Check sheet for the modelled part. Datum: model origin and axes. Units: mm. Face numbers are marked on the shaded views. A direction names the side the tool comes from. Round coordinates to 2 decimals unless told otherwise and drop trailing zeros. Write each loop counter-clockwise with the first axis right and the second up, starting at its lowest first coordinate (ties: lowest second). Pieces come first, ordered by that corner, then holes. Notation, with made-up numbers: (3, 47) -> (31, 47) arc R28 cw to (31, 85) -> close; hole circle Ø5 at (28, -30.75). An arc over 180 degrees is marked (long way). Answer as a JSON object with one key per item and string values. Group by question number.
```python
from build123d import *

# Parameters (mm, degrees)
F0_W           = 76.2
F0_H           = 127
F0_W_2         = 63.5
F0_H_2         = 114.3
F1_DEPTH       = 762
F2_R           = 19.05
F3_DEPTH       = 12.7
F9_W           = 50.8
F9_H           = 127
F9_W_2         = 38.1
F9_H_2         = 114.3
F10_DEPTH      = 381
F12_DEPTH      = 9.525
F12_DEPTH_BACK = 0.254


with BuildPart() as f1:
    # F0 (on Front) → F1 (new body, symmetric)
    with BuildSketch(Plane.XZ):
        with Locations((38.1, 0)):
            Rectangle(F0_W, F0_H)
        with Locations((38.1, 0)):
            Rectangle(F0_W_2, F0_H_2, mode=Mode.SUBTRACT)
    extrude(amount=F1_DEPTH, both=True)

    # F2 (on face) → F3 (join)
    with BuildSketch(Plane.XY.offset(63.5)):
        with BuildLine():
            ThreePointArc((-11.159232, 827.040768), (-65.040768, 827.040768), (-65.040768, 773.159232))
            Line((-65.040768, 773.159232), (11.159232, 696.959232))
            ThreePointArc((11.159232, 696.959232), (65.040768, 696.959232), (65.040768, 750.840768))
            Line((65.040768, 750.840768), (-11.159232, 827.040768))
        make_face()
        with Locations((-38.1, 800.1)):
            Circle(F2_R, mode=Mode.SUBTRACT)
    extrude(amount=F3_DEPTH)

    # F4: F1 across plane


with BuildPart() as f1_1:
    add(f1.part)
    add(f1.part.mirror(Plane.XY))

    # F9 (on face) → F10 (join)
    with BuildSketch(Plane(origin=(-10.770568, 0, 40.196307), x_dir=(0.965926, 0, 0.258819), z_dir=(-0.258819, 0, 0.965926))):
        with Locations((51.938557, 0)):
            Rectangle(F9_W, F9_H)
        with Locations((51.938557, 0)):
            Rectangle(F9_W_2, F9_H_2, mode=Mode.SUBTRACT)
    extrude(amount=F10_DEPTH)

    # F11 (on face) → F12 (join, two sides)
    with BuildSketch(Plane(origin=(74.70331, 0, 20.016692), x_dir=(0, 1, 0), z_dir=(0.965926, 0, 0.258819))) as f12_sk:
        Polygon((0, 422.614279), (-63.5, 422.614279), (-602.764468, 45.017233), (-381.346724, 45.017233), (0, 312.039085), align=None)
    extrude(amount=F12_DEPTH)
    extrude(f12_sk.sketch, amount=-F12_DEPTH_BACK)

    # F13: F1 across face


with BuildPart() as f1_2:
    add(f1_1.part)
    add(f1_1.part.mirror(Plane(origin=(-15.767609, 0, 376.059646), x_dir=(-1, 0, 0), z_dir=(0, 1, 0))))


solid = f1_2.part
```
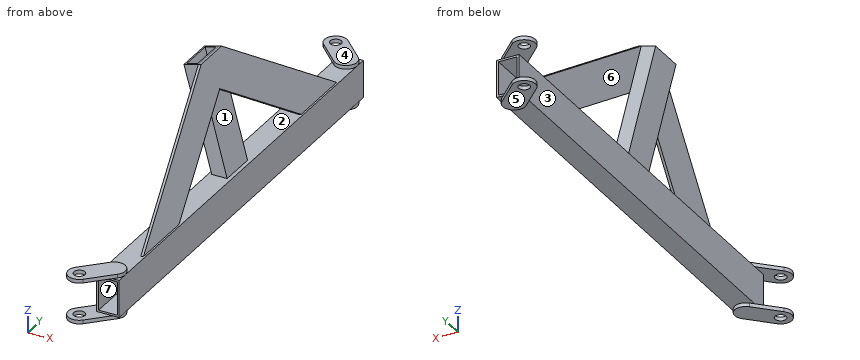
(1) Go/stop test with flat-tipped pins: pin 1 Ø1 at (x, y) = (-2, 400.5) entering from -Z; pin 2 Ø2.5 at (x, z) = (32.5, 51) entering from -Y; pin 3 Ø3 at (x, z) = (29.5, 54.5) entering from +Y; pin 4 Ø4 at (x, y) = (17.5, -357) entering from +Z. Record where each tip stops, or that it passes through.
(2) Section check D-D on x = 38.1. State how many separate pieces and enclosed holes the cut face has, then the cut area to 3 significant figures.
(3) Access from +Z, -Z, +X, -X, +Y, -Y to the whole of each face (thin tool, end or side, straight path). Record for the marked faces 4, 5, 6 and 7.
(4) Section check C-C on y = -639.5. Record the cut outline in (x, z), then the cut area to 3 significant figures.
(5) Release check for a two-part mould opening along Y. For the marked faces 1, 2 and 3 record: pulls with the +Y half, pulls with the -Y half, needs draft (parallel to the pull), parting line crosses it, or undercut.
(6) Scan lines: line 1 along Z through (x, y) = (7, -490); line 2 along X through (y, z) = (-454, -32); line 3 along Y through (x, z) = (-38.1, -69). Record each from-to range of solid material in increasing order.
(7) Section check A-A on z = 161.5. Record the cut outline in (x, y), then the cut area to 3 significant figures.
(8) Section check B-B on z = -23.5. Record the cut outline in (x, y), then the cut area to 3 significant figures.
Data:
{
 "1": {"pin 1": "passes through", "pin 2": "stops at y = -63.5", "pin 3": "stops at y = 63.5", "pin 4": "stops at z = 231"},
 "2": {"separate pieces": "4", "enclosed holes": "1", "area": "44,800 mm²"},
 "3": {"face 4": "+Z, +X, -X, +Y", "face 5": "-Z, +X, -X, +Y, -Y", "face 6": "-X", "face 7": "+Y, -Y"},
 "4": {"outline": "(0, -63.5) -> (76.2, -63.5) -> (76.2, 63.5) -> (0, 63.5) -> close; hole (6.35, -57.15) -> (69.85, -57.15) -> (69.85, 57.15) -> (6.35, 57.15) -> close", "area": "2,420 mm²"},
 "5": {"face 1": "undercut", "face 2": "undercut", "face 3": "needs draft"},
 "6": {"line 1": "z = -63.5 to -57.15, 57.15 to 63.5", "line 2": "x = 0 to 6.35, 69.85 to 76.2", "line 3": "y = -838.2 to -819.15, -781.05 to -746.22, 746.22 to 781.05, 819.15 to 838.2"},
 "7": {"outline": "(-15.8, -63.5) -> (36.79, -63.5) -> (36.79, 63.5) -> (-15.8, 63.5) -> close; (36.53, -457.77) -> (46.65, -461.51) -> (46.65, -240.1) -> (36.53, -236.35) -> close; (36.53, 236.35) -> (46.65, 240.1) -> (46.65, 461.51) -> (36.53, 457.77) -> close; hole (-9.23, -57.15) -> (30.22, -57.15) -> (30.22, 57.15) -> (-9.23, 57.15) -> close", "area": "6,650 mm²"},
 "8": {"outline": "(0, -762) -> (6.35, -762) -> (6.35, 762) -> (0, 762) -> close; (69.85, -762) -> (76.2, -762) -> (76.2, 762) -> (69.85, 762) -> close", "area": "19,400 mm²"}
}
